from build123d import *

# Parameters (mm, degrees)
F0_W      = 65
F0_H      = 156
F0_W_2    = 60
F0_H_2    = 151
F1_DEPTH  = 2
F2_DEPTH  = 7
F3_W      = 10
F3_H      = 2.5
F4_DEPTH  = 5
F5_DEPTH  = 2
F6_R      = 2
F7_R      = 2
F8_W      = 5
F8_H      = 2.5
F8_W_2    = 2.5
F8_H_2    = 5
F9_DEPTH  = 2
F10_DEPTH = 2.5
F11_DEPTH = 2.5
F12_R     = 5


with BuildPart() as f1:
    # F0 (on Top) → F1 (new body)
    with BuildSketch(Plane.XY):
        Rectangle(F0_W, F0_H)
        Rectangle(F0_W_2, F0_H_2, mode=Mode.SUBTRACT)
        Rectangle(F0_W_2, F0_H_2)
    extrude(amount=F1_DEPTH)

    # F0 (on Top) → F2 (join)
    with BuildSketch(Plane.XY):
        Rectangle(F0_W, F0_H)
        Rectangle(F0_W_2, F0_H_2, mode=Mode.SUBTRACT)
    extrude(amount=F2_DEPTH)

    # F3 (on face) → F4 (cut, through all)
    with BuildSketch(Plane.XY.offset(7)):
        with Locations((5, 76.75)):
            Rectangle(F3_W, F3_H)
        with Locations((-5, 76.75)):
            Rectangle(F3_W, F3_H)
    extrude(amount=-F4_DEPTH, mode=Mode.SUBTRACT)

    # F5 (add): a face of the model
    f5_faces = [f1.faces().sort_by_distance(p)[0] for p in [
        (0, -76.31, 7),
    ]]
    extrude(f5_faces, amount=F5_DEPTH)

    # F6
    f6_edges = [f1.edges().sort_by_distance(p)[0] for p in [
        (-32.5, 78, 4.5),
        (32.5, 78, 4.5),
        (32.5, -78, 4.5),
        (-32.5, -78, 4.5),
    ]]
    fillet(f6_edges, radius=F6_R)

    # F7
    f7_edges = [f1.edges().sort_by_distance(p)[0] for p in [
        (-30, 75.5, 5.5),
        (30, 75.5, 5.5),
        (30, -75.5, 5.5),
        (-30, -75.5, 5.5),
    ]]
    fillet(f7_edges, radius=F7_R)

    # F8 (on face) → F9 (cut)
    with BuildSketch(Plane.XY.offset(9)):
        with Locations((2.5, -76.75)):
            Rectangle(F8_W, F8_H)
        with Locations((-2.5, -76.75)):
            Rectangle(F8_W, F8_H)
        with Locations((-31.25, 2.5)):
            Rectangle(F8_W_2, F8_H_2)
        with Locations((-31.25, -2.5)):
            Rectangle(F8_W_2, F8_H_2)
        with Locations((31.25, 2.5)):
            Rectangle(F8_W_2, F8_H_2)
        with Locations((31.25, -2.5)):
            Rectangle(F8_W_2, F8_H_2)
    extrude(amount=-F9_DEPTH, mode=Mode.SUBTRACT)

    # F10 (add): a face of the model
    f10_faces = [f1.faces().sort_by_distance(p)[0] for p in [
        (-10, 76.75, 5.5),
    ]]
    extrude(f10_faces, amount=F10_DEPTH)

    # F11 (add): a face of the model
    f11_faces = [f1.faces().sort_by_distance(p)[0] for p in [
        (10, 76.75, 5.5),
    ]]
    extrude(f11_faces, amount=F11_DEPTH)

    # F12
    f12_edges = [f1.edges().sort_by_distance(p)[0] for p in [
        (7.5, 76.75, 2),
        (-7.5, 76.75, 2),
    ]]
    fillet(f12_edges, radius=F12_R)


solid = f1.part
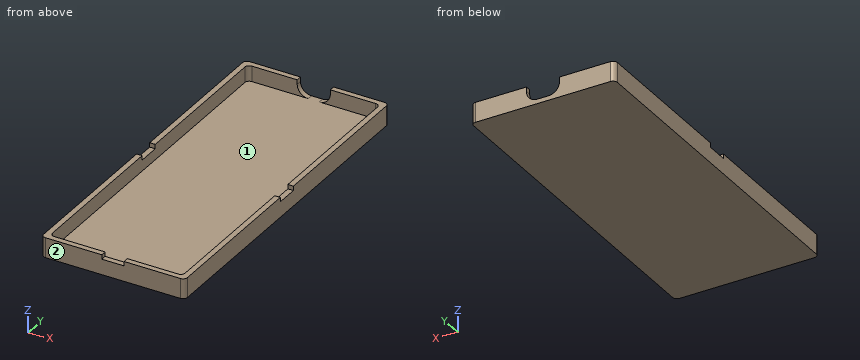
Work out the finished part from the listing and answer in its coordinate system (mm). Face numbers are marked on the shaded views. Round coordinates to 2 decimals unless told otherwise and drop trailing zeros. Write each loop counter-clockwise with the first axis right and the second up, starting at its lowest first coordinate (ties: lowest second). Pieces come first, ordered by that corner, then holes. Notation, with made-up numbers: M 4,51 L 37,51 A14 ccw 37,59 Z; hole C 56.25,84.5 d2. An arc over 180 degrees is marked long. Use a Markdown table: item, result.
1) Determine the mould class of the marked faces 1 and 2 for opening direction X: pulls with the +X half, pulls with the -X half, needs draft (parallel to the pull), parting line crosses it, or undercut.
Taken from the geometry:
| item | result |
|---|---|
| face 1 | undercut |
| face 2 | needs draft |
2) The part is cut by section B-B on y = 8. Give the vertices of the cut face in (x, z).
Taken from the geometry:
| item | result |
|---|---|
| outline | M -32.5,0 L 32.5,0 L 32.5,9 L 30,9 L 30,2 L -30,2 L -30,9 L -32.5,9 Z |
3) The part is cut by section C-C on z = 3.75. Give the vertices of the cut face in (x, y), plus the area to 3 significant figures.
Taken from the geometry:
| item | result |
|---|---|
| outline | M -32.5,-76 A2 ccw -30.5,-78 L 30.5,-78 A2 ccw 32.5,-76 L 32.5,76 A2 ccw 30.5,78 L 6.3,78 L 6.3,75.5 L 28,75.5 A2 cw 30,73.5 L 30,-73.5 A2 cw 28,-75.5 L -28,-75.5 A2 cw -30,-73.5 L -30,73.5 A2 cw -28,75.5 L -6.3,75.5 L -6.3,78 L -30.5,78 A2 ccw -32.5,76 Z |
| area | 1,050 mm2 |
4) Consider line 1 (X direction, y = -64, z = 6.25); line 2 (Y direction, x = -25, z = 3.75); line 3 (Z direction, x = -17, y = -19). Determine where each line is inside the solid, lowest interval first. Write a range as [from, to].
Taken from the geometry:
| item | result |
|---|---|
| line 1 | x = [-32.5, -30], [30, 32.5] |
| line 2 | y = [-78, -75.5], [75.5, 78] |
| line 3 | z = [0, 2] |
5) The part is cut by section A-A on x = -17. Give the vertices of the cut face in (y, z), plus the area to 3 significant figures.
Taken from the geometry:
| item | result |
|---|---|
| outline | M -78,0 L 78,0 L 78,9 L 75.5,9 L 75.5,2 L -75.5,2 L -75.5,9 L -78,9 Z |
| area | 347 mm2 |
6) Flat-ended cylindrical pins translate along their axes: pin 1 (1.6 mm diameter, centred on y = -76.5, z = 8.5, fed in from +X); pin 2 (18 mm diameter, centred on x = -9.5, y = 7, fed in from +Z); pin 3 (0.6 mm diameter, centred on x = -31, z = 8, fed in from +Y); pin 4 (0.8 mm diameter, centred on x = 30.5, y = 2, fed in from +Z). Find the tip coordinate at first contact, or state that the pin passes through.
Taken from the geometry:
| item | result |
|---|---|
| pin 1 | stops at x = 32.5 |
| pin 2 | stops at z = 2 |
| pin 3 | stops at y = 77.99 |
| pin 4 | stops at z = 7 |
